Here's how the part is built. I have some questions about the finished solid (model axes, mm). A direction names the side the tool comes from. Round coordinates to 2 decimals unless told otherwise and drop trailing zeros. Loops run counter-clockwise (first coordinate to the right, second up) from the corner with the lowest first, then second, coordinate; pieces in that order, holes last. Notation, with made-up numbers: (-16, -19) - (-8, -19) arc R20 cw to (-8, -15) - close; hole circle Ø4 at (-5, -40). An arc over 180 degrees is marked (long way). Answer as a JSON object with one key per item and string values. Group by question number.
1) I want a section at B-B, the plane z = 4.25. Please give me the cut outline in (x, y) (3 decimals), then the cut area to 3 significant figures.
2) If we mould it in two halves opening along X, with no side actions, what happens to faces 4 (the face through (-97.795, -3.178, 1.61)), 5 (the face through (-42.601, -35.853, 1.565)), 6 (the face through (-1, 127.701, 3))? For each: pulls with the +X half, pulls with the -X half, needs draft (parallel to the pull), parting line crosses it, or undercut.
3) Will these pins go through, and if not, where does the flat tip stop? P1, Ø1, axis at x = 26.5, z = 4, coming from the -Y side; P2, Ø5, axis at x = -38.5, y = -103.5, coming from the -Z side.
4) I want a section at C-C, the plane x = 17.5. Please give me the cut outline in (y, z) (3 decimals).
5) I want a section at A-A, the plane x = 93.98. Please give me the cut outline in (y, z) (3 decimals), then the cut area to 3 significant figures.
6) Which directions (+Z, -Z, +X, -X, +Y, -Y) give clear straight access to the entire face, cutting with the end or side of a thin tool? Please do faces 1 (the face through (1, -6, 3.175)), 2 (the face through (-31.059, -93.353, 1.565)), 3 (the face through (86.35, -120.52, 4.74)).
7) If I drill on line 1 along Y through (x, z) = (-93.98, 4.7); line 2 along Y through (x, z) = (-93.98, 1.7); line 3 along X through (y, z) = (-81, 4.5) (3 decimals), over which ranges is the centre line in solid material (lowest first)? Write a range as [from, to].
from build123d import *

# Parameters (mm, degrees)
SKETCH1_W                   = 104.775
SKETCH1_H                   = 251.46
BOSS_EXTRUDE2_DEPTH         = 3.175
CUTOUT_FILLETS_R            = 5
SKETCH2_W                   = 22.225
SKETCH2_H                   = 251.46
SKETCH2_R                   = 8
BOSS_EXTRUDE3_DEPTH         = 3.175
SKETCH3_R                   = 3
SKETCH3_R_2                 = 4
CUT_EXTRUDE1_DEPTH          = 30
CUTOUT_FILLETS_OF_MIRROR2_R = 5
SKETCH4_W                   = 209.55
SKETCH4_H                   = 6.35
BOSS_EXTRUDE4_DEPTH         = 10.16


with BuildPart() as part:
    # Sketch1 → Boss-Extrude2 (new body)
    with BuildSketch(Plane.XY):
        with Locations((52.3875, -8.189050142)):
            Rectangle(SKETCH1_W, SKETCH1_H)
        Polygon((4, 104.466937315), (4, 59.163810249), (62.035275472, 104.466937315), align=None, mode=Mode.SUBTRACT)
        Polygon((69.66, 100.270064381), (11.624724528, 54.966937315), (69.66, 54.966937315), align=None, mode=Mode.SUBTRACT)
        Polygon((11.624724528, 46.966937315), (69.66, 46.966937315), (69.66, 1.663810249), align=None, mode=Mode.SUBTRACT)
        Polygon((62.035275472, -2.533062685), (4, 42.770064381), (4, -2.533062685), align=None, mode=Mode.SUBTRACT)
        Polygon((4, -10.533062685), (62.035275472, -10.533062685), (4, -55.836189751), align=None, mode=Mode.SUBTRACT)
        Polygon((69.66, -14.729935619), (11.624724528, -60.033062685), (69.66, -60.033062685), align=None, mode=Mode.SUBTRACT)
        Polygon((11.624724528, -68.033062685), (69.66, -68.033062685), (69.66, -113.336189751), align=None, mode=Mode.SUBTRACT)
        Polygon((4, -117.533062685), (4, -72.229935619), (62.035275472, -117.533062685), align=None, mode=Mode.SUBTRACT)
    boss_extrude2 = extrude(amount=BOSS_EXTRUDE2_DEPTH)

    # Cutout_Fillets
    cutout_fillets_edges = [part.edges().sort_by_distance(p)[0] for p in [
        (62.035275472, 104.466937315, 1.5875),
        (4, 104.466937315, 1.5875),
        (4, 59.163810249, 1.5875),
        (69.66, 54.966937315, 1.5875),
        (69.66, 100.270064381, 1.5875),
        (11.624724528, 54.966937315, 1.5875),
        (11.624724528, 46.966937315, 1.5875),
        (69.66, 1.663810249, 1.5875),
        (69.66, 46.966937315, 1.5875),
        (4, -2.533062685, 1.5875),
        (62.035275472, -2.533062685, 1.5875),
        (4, 42.770064381, 1.5875),
        (4, -10.533062685, 1.5875),
        (4, -55.836189751, 1.5875),
        (62.035275472, -10.533062685, 1.5875),
        (69.66, -60.033062685, 1.5875),
        (69.66, -14.729935619, 1.5875),
        (11.624724528, -60.033062685, 1.5875),
        (11.624724528, -68.033062685, 1.5875),
        (69.66, -113.336189751, 1.5875),
        (69.66, -68.033062685, 1.5875),
        (4, -117.533062685, 1.5875),
        (62.035275472, -117.533062685, 1.5875),
        (4, -72.229935619, 1.5875),
    ]]
    fillet(cutout_fillets_edges, radius=CUTOUT_FILLETS_R)

    # Sketch2 → Boss-Extrude3 (add)
    with BuildSketch(Plane.XY.offset(3.175)):
        with Locations((93.6625, -8.189050142)):
            Rectangle(SKETCH2_W, SKETCH2_H)
        with Locations(Location((93.98, -118.115286613, 0), (0, 0, 180))):
            Circle(SKETCH2_R, mode=Mode.SUBTRACT)
        with Locations(Location((93.98, -4.379050142, 0), (0, 0, 180))):
            Circle(SKETCH2_R, mode=Mode.SUBTRACT)
        with Locations(Location((93.98, 105.540949858, 0), (0, 0, 180))):
            Circle(SKETCH2_R, mode=Mode.SUBTRACT)
    boss_extrude3 = extrude(amount=BOSS_EXTRUDE3_DEPTH)

    # Sketch3 → Cut-Extrude1 (cut)
    with BuildSketch(Plane.XY.offset(6.35)):
        with Locations((93.98, 105.540949858)):
            Circle(SKETCH3_R)
        with Locations((93.98, -4.379050142)):
            Circle(SKETCH3_R_2)
        with Locations((93.98, -118.115286613)):
            Circle(SKETCH3_R)
    cut_extrude1 = extrude(amount=-CUT_EXTRUDE1_DEPTH, mode=Mode.SUBTRACT)

    # Mirror2: Boss-Extrude2, Boss-Extrude3, Cut-Extrude1 across Right Plane
    add(boss_extrude2.mirror(Plane(origin=(0, 0, 0), x_dir=(0, 0, -1), z_dir=(1, 0, 0))))
    add(boss_extrude3.mirror(Plane(origin=(0, 0, 0), x_dir=(0, 0, -1), z_dir=(1, 0, 0))))
    add(cut_extrude1.mirror(Plane(origin=(0, 0, 0), x_dir=(0, 0, -1), z_dir=(1, 0, 0))), mode=Mode.SUBTRACT)

    # Cutout_Fillets of Mirror2
    cutout_fillets_of_mirror2_edges = [part.edges().sort_by_distance(p)[0] for p in [
        (-62.035275472, 104.466937315, 1.5875),
        (-4, 104.466937315, 1.5875),
        (-4, 59.163810249, 1.5875),
        (-69.66, 54.966937315, 1.5875),
        (-69.66, 100.270064381, 1.5875),
        (-11.624724528, 54.966937315, 1.5875),
        (-11.624724528, 46.966937315, 1.5875),
        (-69.66, 1.663810249, 1.5875),
        (-69.66, 46.966937315, 1.5875),
        (-4, -2.533062685, 1.5875),
        (-62.035275472, -2.533062685, 1.5875),
        (-4, 42.770064381, 1.5875),
        (-4, -10.533062685, 1.5875),
        (-4, -55.836189751, 1.5875),
        (-62.035275472, -10.533062685, 1.5875),
        (-69.66, -60.033062685, 1.5875),
        (-69.66, -14.729935619, 1.5875),
        (-11.624724528, -60.033062685, 1.5875),
        (-11.624724528, -68.033062685, 1.5875),
        (-69.66, -113.336189751, 1.5875),
        (-69.66, -68.033062685, 1.5875),
        (-4, -117.533062685, 1.5875),
        (-62.035275472, -117.533062685, 1.5875),
        (-4, -72.229935619, 1.5875),
    ]]
    fillet(cutout_fillets_of_mirror2_edges, radius=CUTOUT_FILLETS_OF_MIRROR2_R)

    # Sketch4 → Boss-Extrude4 (add)
    with BuildSketch(Plane(origin=(0, 117.540949858, 0), x_dir=(1, 0, 0), z_dir=(0, 1, 0))):
        with Locations((0, -3.175)):
            Rectangle(SKETCH4_W, SKETCH4_H)
    extrude(amount=BOSS_EXTRUDE4_DEPTH)


solid = part.part
Outcome:
{
 "1": {"outline": "(-104.775, -133.919) - (-82.55, -133.919) - (-82.55, 117.541) - (82.55, 117.541) - (82.55, -133.919) - (104.775, -133.919) - (104.775, 127.701) - (-104.775, 127.701) - close; hole circle Ø16 at (-93.98, -118.115); hole circle Ø16 at (-93.98, -4.379); hole circle Ø16 at (-93.98, 105.541); hole circle Ø16 at (93.98, -118.115); hole circle Ø16 at (93.98, -4.379); hole circle Ø16 at (93.98, 105.541)", "area": "12,100 mm^2"},
 "2": {"face 4": "undercut", "face 5": "undercut", "face 6": "needs draft"},
 "3": {"P1": "y = 117.54", "P2": "through"},
 "4": {"outline": "(-133.919, 0) - (-117.533, 0) - (-117.533, 3.175) - (-133.919, 3.175) - close; (-82.768, 0) - (-45.298, 0) - (-45.298, 3.175) - (-82.768, 3.175) - close; (-10.533, 0) - (-2.533, 0) - (-2.533, 3.175) - (-10.533, 3.175) - close; (32.232, 0) - (69.702, 0) - (69.702, 3.175) - (32.232, 3.175) - close; (104.467, 0) - (127.701, 0) - (127.701, 6.35) - (117.541, 6.35) - (117.541, 3.175) - (104.467, 3.175) - close"},
 "5": {"outline": "(-133.919, 0) - (-121.115, 0) - (-121.115, 3.175) - (-126.115, 3.175) - (-126.115, 6.35) - (-133.919, 6.35) - close; (-115.115, 0) - (-8.379, 0) - (-8.379, 3.175) - (-12.379, 3.175) - (-12.379, 6.35) - (-110.115, 6.35) - (-110.115, 3.175) - (-115.115, 3.175) - close; (-0.379, 0) - (102.541, 0) - (102.541, 3.175) - (97.541, 3.175) - (97.541, 6.35) - (3.621, 6.35) - (3.621, 3.175) - (-0.379, 3.175) - close; (108.541, 0) - (127.701, 0) - (127.701, 6.35) - (113.541, 6.35) - (113.541, 3.175) - (108.541, 3.175) - close", "area": "1,450 mm^2"},
 "6": {"face 1": "+Z, -Y", "face 2": "+Z, -Z", "face 3": "+Z"},
 "7": {"line 1": "[-133.92, -126.12], [-110.12, -12.38], [3.62, 97.54], [113.54, 127.7]", "line 2": "[-133.92, -121.12], [-115.12, -8.38], [-0.38, 102.54], [108.54, 127.7]", "line 3": "[-104.775, -82.55], [82.55, 104.775]"}
}
